Work out the finished part from the listing and answer in its coordinate system (mm). A direction names the side the tool comes from. Coordinates: 2 decimals unless noted, no trailing zeros. Write each loop counter-clockwise with the first axis right and the second up, starting at its lowest first coordinate (ties: lowest second). Pieces come first, ordered by that corner, then holes. Notation, with made-up numbers: (89.25, 63.5) - (97.25, 63.5) arc R9 ccw to (97.25, 78.5) - close; hole circle Ø8 at (-4, -15). An arc over 180 degrees is marked (long way). Use a Markdown table: item, result. Add a question column.
(1) The part is cut by section C-C, the plane z = -110. Give the vertices of the cut face in (x, y), then the cut area to 3 significant figures.
(2) For a pull along Z with two mould halves and no side action, classify faces 4 (the face through (-42, 2, -35.477)), 5 (the face through (-39, 0, -90)), 6 (the face through (-116.944, 6.252, -57.338)) as released by +Z, released by -Z, zero draft, split by the parting line, or undercut.
(3) Find the intervals of material crossed by line 1 (Z direction, x = -59, y = 2); line 2 (X direction, y = 3.25, z = -104.5); line 3 (Y direction, x = 25, z = -71), in increasing order. Write a range as from..to.
(4) A tool of negligible diameter and unlimited length cuts with its end or side. For faces 1 (the face through (29.89, 6.25, -55.33)), 2 (the face through (-112, 7.54, -104)), 3 (the face through (-40, 3, -81.827)), from which of +Z, -Z, +X, -X, +Y, -Y can it reach the whole face along a straight path? Write none if from no direction.
(5) The part is cut by section D-D, the plane x = -107.5. Give the vertices of the cut face in (y, z), then the cut area to 3 significant figures.
(6) The part is cut by section B-B, the plane y = 6.25. Give the vertices of the cut face in (x, z) (3 decimals).
(7) The part is cut by section A-A, the plane x = -19. Give the vertices of the cut face in (y, z), then the cut area to 4 significant figures.
(8) Given pin 1 Ø1.6 at (x, z) = (32.23, -57.48) entering from +Y; pin 2 Ø4 at (x, z) = (-44.5, -76) entering from +Y, each flat-ended and moving along its own axis, determine where each tip first touches the part or whether it passes through.
Autodesk Inventor part; units mm, degrees
ref_plane "YZ Plane" through (0, 0, 0) normal (1, 0, 0) x (0, 1, 0)
ref_plane "XZ Plane" through (0, 0, 0) normal (0, 1, 0) x (-1, 0, 0)
ref_plane "XY Plane" through (0, 0, 0) normal (0, 0, 1) x (1, 0, 0)
sketch "Sketch1" plane through (0, 0, 0) normal (0, 1, 0) x (-1, 0, 0)
  circle A0 centre (113.7717, -57.4772) radius 1.35
  circle A1 centre (113.7717, -103.4772) radius 1.35
  circle A2 centre (-32.2283, -57.4772) radius 1.35
  circle A3 centre (-32.2283, -103.4772) radius 1.35
  line L0 (140.7717, -35.4772) -> (-59.2283, -35.4772)
  line L1 (-59.2283, -35.4772) -> (-59.2283, -125.4772)
  line L2 (-59.2283, -125.4772) -> (140.7717, -125.4772)
  line L3 (140.7717, -125.4772) -> (140.7717, -35.4772)
  point P0 (0, 0)
  point P1 (140.7717, -80.4772)
  dimension "d2" = 2.7
  dimension "d3" = 2.7
  dimension "d4" = 2.7
  dimension "d5" = 2.7
  dimension "d6" = 200
  dimension "d7" = 90
extrude "Extrusion1" add sketch "Sketch1" along normal blind 5
sketch "Sketch2" plane through (0, 5, 0) normal (0, 1, 0) x (1, 0, 0)
  circle A0 centre (-72.5219, 80.4772) radius 1.35
  circle A1 centre (-9.0219, 80.4772) radius 1.35
  circle A2 centre (-40.7719, 80.4772) radius 1.35
  line L0 (-140.7717, 125.4772) -> (-140.7717, 35.4772)
  point P0 (0, 0)
  point P1 (-140.7717, 80.4772)
  dimension "d12" = 2.7
  dimension "d13" = 2.7
  dimension "d14" = 63.5
  dimension "d15" = 2.7
  dimension "d16" = 31.75
  dimension "d22" = 68.2498
extrude "Extrusion2" cut sketch "Sketch2" against normal blind 11.35
sketch "Sketch3" plane through (0, 5, 0) normal (0, 1, 0) x (1, 0, 0)
  circle A0 centre (-113.7717, 57.4772) radius 1.35
  circle A1 centre (-113.7717, 57.4772) radius 3.175
  circle A2 centre (-113.7717, 57.4772) radius 1.35
  circle A3 centre (-113.7717, 103.4772) radius 1.35
  circle A4 centre (-113.7717, 103.4772) radius 1.35
  circle A5 centre (-113.7717, 103.4772) radius 3.175
  circle A6 centre (32.2283, 103.4772) radius 1.35
  circle A7 centre (32.2283, 103.4772) radius 1.35
  circle A8 centre (32.2283, 103.4772) radius 3.175
  circle A9 centre (32.2283, 57.4772) radius 1.35
  circle A10 centre (32.2283, 57.4772) radius 1.35
  circle A11 centre (32.2283, 57.4772) radius 3.175
  point P0 (0, 0)
  dimension "d25" = 6.35
  dimension "d26" = 6.35
  dimension "d27" = 6.35
  dimension "d28" = 6.35
extrude "Extrusion3" add sketch "Sketch3" along normal blind 2.54 contours A0 | A1 | A3 | A5 | A6 | A8 | A9 | A11
sketch "Sketch4" plane through (-113.7717, 7.54, -57.4772) normal (0, 1, 0) x (1, 0, 0)
  circle A0 centre (0, 0) radius 1.35
  circle A1 centre (0, 0) radius 1.35
  circle A2 centre (0, 46) radius 1.35
  circle A3 centre (0, 46) radius 1.35
  circle A4 centre (146, 46) radius 1.35
  circle A5 centre (146, 46) radius 1.35
  circle A6 centre (146, 0) radius 3.175
  circle A7 centre (146, 0) radius 1.35
  point P0 (113.7717, -57.4772)
  dimension "d31" = 2.7
  dimension "d32" = 2.7
  dimension "d33" = 2.7
  dimension "d34" = 2.7
extrude "Extrusion4" cut sketch "Sketch4" against normal blind 21.59 contours A0 | A2 | A4 | A7
sketch "Sketch5" plane through (0, 5, 0) normal (0, 1, 0) x (1, 0, 0)
  circle A0 centre (-72.5219, 80.4772) radius 1.35
  circle A1 centre (-9.0219, 80.4772) radius 1.35
  line L0 (-72.5219, 79.1272) -> (-9.0219, 79.1272)
  line L1 (-9.0219, 79.1272) -> (-9.0219, 81.8272)
  line L2 (-9.0219, 81.8272) -> (-72.5219, 81.8272)
  line L3 (-72.5219, 81.8272) -> (-72.5219, 79.1272)
  line L4 (-72.5219, 81.8272) -> (-81.2922, 81.8272)
  line L5 (-81.2922, 81.8272) -> (-81.2922, 79.1272)
  line L6 (-81.2922, 79.1272) -> (-72.5219, 79.1272)
  line L7 (-72.5219, 79.1272) -> (-72.5219, 81.8272)
  line L8 (-9.0219, 81.8272) -> (-0.2589, 81.8272)
  line L9 (-0.2589, 81.8272) -> (-0.2589, 79.1272)
  line L10 (-0.2589, 79.1272) -> (-9.0219, 79.1272)
  line L11 (-9.0219, 79.1272) -> (-9.0219, 81.8272)
  circle A2 centre (-81.2922, 80.4772) radius 1.35
  circle A3 centre (-0.2589, 80.4772) radius 1.35
  point P0 (0, 0)
  dimension "d37" = 8.763
  dimension "d38" = 8.7702
extrude "Extrusion5" cut sketch "Sketch5" against normal up to surface (5 mm away) contours A0 L3 | A0 L2 A1 L0 | L3 A0 | A0 L6 A2 L4 | L8 A3 L10 A1 | A2 L5 | L5 A2 | A3 L9 | L9 A3
properties part number "battery holder v2 mount"
Model answer:
| question | item | result |
|---|---|---|
| 1 | outline | (-140.77, 0) - (59.23, 0) - (59.23, 5) - (-140.77, 5) - close |
| 1 | area | 1,000 mm^2 |
| 2 | face 4 | released by +Z |
| 2 | face 5 | zero draft |
| 2 | face 6 | undercut |
| 3 | line 1 | -125.48..-81.83, -79.13..-35.48 |
| 3 | line 2 | -140.77..-114.65, -112.89..31.35, 33.11..59.23 |
| 3 | line 3 | 0..5 |
| 4 | face 1 | +Y |
| 4 | face 2 | +Z, -Z, +X, -X, +Y |
| 4 | face 3 | +Y, -Y |
| 5 | outline | (0, -125.48) - (5, -125.48) - (5, -35.48) - (0, -35.48) - close |
| 5 | area | 450 mm^2 |
| 6 | outline | circle Ø6.35 at (-113.772, -103.477); circle Ø6.35 at (-113.772, -57.477); circle Ø6.35 at (32.228, -103.477); circle Ø6.35 at (32.228, -57.477); hole circle Ø2.7 at (-113.772, -103.477); hole circle Ø2.7 at (-113.772, -57.477); hole circle Ø2.7 at (32.228, -103.477); hole circle Ø2.7 at (32.228, -57.477) |
| 7 | outline | (0, -125.48) - (5, -125.48) - (5, -81.83) - (0, -81.83) - close; (0, -79.13) - (5, -79.13) - (5, -35.48) - (0, -35.48) - close |
| 7 | area | 436.5 mm^2 |
| 8 | pin 1 | through |
| 8 | pin 2 | y = 5 |
